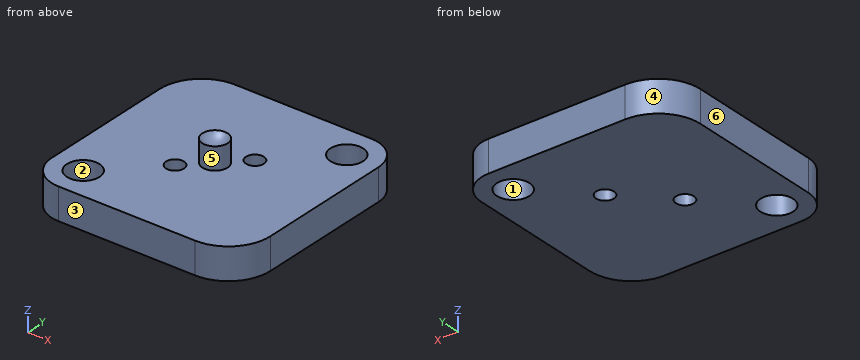
```python
from build123d import *

# Parameters (mm, degrees)
SKETCH1_W           = 100
SKETCH1_H           = 100
BOSS_EXTRUDE1_DEPTH = 15
SKETCH2_R           = 7.75
CUT_EXTRUDE1_DEPTH  = 73.284161474
SKETCH5_R           = 6
BOSS_EXTRUDE6_DEPTH = 10.5
SKETCH6_R           = 4.25
CUT_EXTRUDE3_DEPTH  = 73.284161474
FILLET1_R           = 20
FILLET2_R           = 15
DOME2_FACE_RADIUS   = 6
DOME2_HEIGHT        = 3


with BuildPart() as part:
    # Sketch1 → Boss-Extrude1 (new body)
    with BuildSketch(Plane.XY):
        Rectangle(SKETCH1_W, SKETCH1_H)
    extrude(amount=BOSS_EXTRUDE1_DEPTH)

    # Sketch2 → Cut-Extrude1 (cut, through all)
    with BuildSketch(Plane.XY.offset(15)):
        with Locations((35, 35)):
            Circle(SKETCH2_R)
        with Locations(Location((-35, -35, 0), (0, 0, 180))):
            Circle(SKETCH2_R)
    extrude(amount=-CUT_EXTRUDE1_DEPTH, mode=Mode.SUBTRACT)

    # Sketch5 → Boss-Extrude6 (add)
    with BuildSketch(Plane.XY.offset(15)):
        with Locations(Location((0, 0, 0), (0, 0, 180))):
            Circle(SKETCH5_R)
    extrude(amount=BOSS_EXTRUDE6_DEPTH)

    # Sketch6 → Cut-Extrude3 (cut, through all)
    with BuildSketch(Plane.XY.offset(15)):
        with Locations((10.606601718, 10.606601718)):
            Circle(SKETCH6_R)
        with Locations(Location((-10.606601718, -10.606601718, 0), (0, 0, 180))):
            Circle(SKETCH6_R)
    extrude(amount=-CUT_EXTRUDE3_DEPTH, mode=Mode.SUBTRACT)

    # Fillet1
    fillet1_edges = [part.edges().sort_by_distance(p)[0] for p in [
        (-50, 50, 7.5),
        (50, -50, 7.5),
    ]]
    fillet(fillet1_edges, radius=FILLET1_R)

    # Fillet2
    fillet2_edges = [part.edges().sort_by_distance(p)[0] for p in [
        (50, 50, 7.5),
        (-50, -50, 7.5),
    ]]
    fillet(fillet2_edges, radius=FILLET2_R)

    # Dome2: a dome of height H over a round flat face of radius A is a cap of a sphere of radius (A * A + H * H) / (2 * H)
    dome2_r = (DOME2_FACE_RADIUS * DOME2_FACE_RADIUS + DOME2_HEIGHT * DOME2_HEIGHT) / (2 * DOME2_HEIGHT)
    dome2_base = Plane((0, 0, 25.5), z_dir=(0, 0, -1))
    with Locations(dome2_base.offset(DOME2_HEIGHT - dome2_r)):
        dome2_ball = Sphere(dome2_r, mode=Mode.PRIVATE)
    add(split(dome2_ball, bisect_by=dome2_base, keep=Keep.TOP, mode=Mode.PRIVATE), mode=Mode.SUBTRACT)


solid = part.part
```
Part model, mm, in its own coordinate system. Face numbers are marked on the shaded views. A direction names the side the tool comes from. Give positions to 0.01 mm unless a question says otherwise; leave off trailing zeros. Write each loop counter-clockwise with the first axis right and the second up, starting at its lowest first coordinate (ties: lowest second). Pieces come first, ordered by that corner, then holes. Notation, with made-up numbers: (89, 43.5) -> (101, 43.5) arc R19 ccw to (101, 55.5) -> close; hole circle Ø2 at (1.5, 19.25). An arc over 180 degrees is marked (long way). Put each result on its own line as item: value. Start each with the question number.
Item 1: Cut at D-D (z = 12.75). List the corners of the cut face in (x, y).
Item 2: Pull direction Y, two halves, no side cores. Call the marked faces 1, 2, 3 and 4: pulls with the +Y half, pulls with the -Y half, needs draft (parallel to the pull), parting line crosses it, or undercut.
Item 3: Which spindle directions (+Z, -Z, +X, -X, +Y, -Y) get a long thin tool onto all of the face, cutting with end or side? Do the marked faces 5 and 6. Say none if no direction does.
Item 4: Pin check, flat tip, straight feed: pin 1 Ø7.5 at (x, y) = (10.61, 10.61) entering from +Z. Stop position of the tip, or through.
Item 5: Cut at C-C (y = -37.5). List the corners of the cut face in (x, z).
Item 6: Wall check: L1, parallel to Y at x = -35, z = 10.25; L2, parallel to Y at x = 35, z = 6.25; L3, parallel to Z at x = 4, y = 37.5. Give the ranges that are in metal, low to high. Write a range as [from, to].
Item 7: Cut at A-A (y = 0). List the corners of the cut face in (x, z), then the cut area to 3 significant figures.
Answer list:
1. outline: (-50, -35) arc R15 ccw to (-35, -50) -> (30, -50) arc R20 ccw to (50, -30) -> (50, 35) arc R15 ccw to (35, 50) -> (-30, 50) arc R20 ccw to (-50, 30) -> close; hole circle Ø15.5 at (-35, -35); hole circle Ø8.5 at (-10.61, -10.61); hole circle Ø8.5 at (10.61, 10.61); hole circle Ø15.5 at (35, 35)
2. face 1: undercut
2. face 2: undercut
2. face 3: pulls with the -Y half
2. face 4: pulls with the +Y half
3. face 5: +Z
3. face 6: +Z, -Z, -X, +Y, -Y
4. pin 1: passes through
5. outline: (-49.79, 0) -> (-42.34, 0) -> (-42.34, 15) -> (-49.79, 15) -> close; (-27.66, 0) -> (48.54, 0) -> (48.54, 15) -> (-27.66, 15) -> close
6. L1: y = [-50, -42.75], [-27.25, 49.36]
6. L2: y = [-49.36, 27.25], [42.75, 50]
6. L3: z = [0, 15]
7. outline: (-50, 0) -> (50, 0) -> (50, 15) -> (6, 15) -> (6, 25.5) arc R7.5 cw to (-6, 25.5) -> (-6, 15) -> (-50, 15) -> close
7. area: 1,600 mm2
